Read the model definition and answer for the solid it produces. Units are mm, in the model's axes. A direction names the side the tool comes from. Coordinates: 2 decimals unless noted, no trailing zeros. Order: outer loops, then holes, each group sorted by start corner. A loop starts at its lowest first (then second) coordinate and runs counter-clockwise, first axis right, second up. Notation, with made-up numbers: M 72.25,-7 L 92.25,-7 A29 cw 92.25,22 Z; hole C 78,-25.75 d5. An arc over 180 degrees is marked long. Use a Markdown table: item, result. Add a question column.
1) Find the intervals of material crossed by probe 1 along X at (y, z) = (13.5, 21); probe 2 along Y at (x, z) = (12.5, 61.5), in increasing order. Write a range as [from, to].
2) The mould has two halves that part along X. Classify faces 1 (the face through (50.8, 13, 50)), 2 (the face through (26, 25.4, 50)), 3 (the face through (25, 1.588, 50)): released by +X, released by -X, zero draft, split by the parting line, or undercut.
3) Find section B-B on x = 44. Write down the section's boundary in (y, z).
4) Find section C-C on z = 75. Write down the section's boundary in (x, y).
5) Each of these flat-tipped pins is pushed along its axis until it touches: pin 1 Ø5 at (x, y) = (39, 22.5) entering from +Z; pin 2 Ø4 at (x, y) = (33.5, 21.5) entering from +Z. Where does it stop, or does it pass through?
6) Find section A-A on y = 21.5. Write down the section's boundary in (x, z), plus the area to 3 significant figures.
7) For faces 4 (the face through (26, 23.812, 50)), 5 (the face through (23, 1, 101.6)), determine the directions among +Z, -Z, +X, -X, +Y, -Y from which every point of the face is accessible in a straight line to the end or side of a thin tool.
Autodesk Inventor part; units mm, degrees
ref_plane "YZ Plane" through (0, 0, 0) normal (1, 0, 0) x (0, 1, 0)
ref_plane "XZ Plane" through (0, 0, 0) normal (0, 1, 0) x (-1, 0, 0)
ref_plane "XY Plane" through (0, 0, 0) normal (0, 0, 1) x (1, 0, 0)
sketch "Sketch1" plane through (0, 0, 0) normal (0, 0, 1) x (1, 0, 0)
  line L0 (0, 0) -> (50.8, 0)
  line L1 (50.8, 0) -> (50.8, 25.4)
  line L2 (50.8, 25.4) -> (0, 25.4)
  line L3 (0, 25.4) -> (0, 0)
  dimension "d0" = 50.8
  dimension "d1" = 25.4
extrude "Extrusion1" add sketch "Sketch1" along normal blind 101.6
shell "Shell1" thickness 1.5875 removed faces 2 at (16.9333, 8.4667, 0) at (16.9333, 8.4667, 101.6)
equation "\"d2\" = Length"
equation "\"Length\" = 101.6"
properties part number "standoff option1"
Check result:
| question | item | result |
|---|---|---|
| 1 | probe 1 | x = [0, 1.59], [49.21, 50.8] |
| 1 | probe 2 | y = [0, 1.59], [23.81, 25.4] |
| 2 | face 1 | released by +X |
| 2 | face 2 | zero draft |
| 2 | face 3 | undercut |
| 3 | outline | M 0,0 L 1.59,0 L 1.59,101.6 L 0,101.6 Z; M 23.81,0 L 25.4,0 L 25.4,101.6 L 23.81,101.6 Z |
| 4 | outline | M 0,0 L 50.8,0 L 50.8,25.4 L 0,25.4 Z; hole M 1.59,1.59 L 49.21,1.59 L 49.21,23.81 L 1.59,23.81 Z |
| 5 | pin 1 | stops at z = 101.6 |
| 5 | pin 2 | passes through |
| 6 | outline | M 0,0 L 1.59,0 L 1.59,101.6 L 0,101.6 Z; M 49.21,0 L 50.8,0 L 50.8,101.6 L 49.21,101.6 Z |
| 6 | area | 323 mm2 |
| 7 | face 4 | +Z, -Z |
| 7 | face 5 | +Z, +X, -X, +Y, -Y |
